CAD build for the part. Positions are in the model's coordinates, mm. Coordinates: 2 decimals unless noted, no trailing zeros. Loops run counter-clockwise (first coordinate to the right, second up) from the corner with the lowest first, then second, coordinate; pieces in that order, holes last. Notation, with made-up numbers: (33.5, 73) -> (79.5, 73) arc R31 ccw to (79.5, 102) -> close; hole circle Ø8 at (53.25, 36). An arc over 180 degrees is marked (long way). Answer as CSV lines item,"result". Start each with the question number.
from build123d import *

# Parameters (mm, degrees)
EXTRUDE_1_DEPTH = 7
EXTRUDE_2_DEPTH = 9


with BuildPart() as part:
    # 草图1 → 凸台-拉伸1 (new body)
    with BuildSketch(Plane(origin=(0, 0, 0), x_dir=(1, 0, 0), z_dir=(0, 1, 0))):
        Polygon((-112.559101124, 19.665498127), (-92.311400749, -15.404547658), (-72.063700375, -50.474593443), (-31.568299625, -50.474593443), (8.927101124, -50.474593443), (29.174801498, -15.404547658), (49.422501873, 19.665498127), (29.174801498, 54.735543912), (8.927101124, 89.805589698), (-31.568299625, 89.805589698), (-72.063700375, 89.805589698), (-92.311400749, 54.735543912), align=None)
        Polygon((-68.02224849, 86.805589698), (-34.455050971, 86.805589698), (-51.23864973, 57.735543912), align=None, mode=Mode.SUBTRACT)
        Polygon((8.349750855, 84.805589697), (24.555999345, 56.735543912), (-7.856497635, 56.735543912), align=None, mode=Mode.SUBTRACT)
        Polygon((-9.011198174, 52.735543912), (8.349750855, 22.665498127), (25.710699883, 52.735543912), align=None, mode=Mode.SUBTRACT)
        Polygon((28.597451229, 49.735543912), (44.803699719, 21.665498127), (12.39120274, 21.665498127), align=None, mode=Mode.SUBTRACT)
        Polygon((11.2365022, 17.665498127), (28.02010096, -11.404547658), (44.803699719, 17.665498127), align=None, mode=Mode.SUBTRACT)
        Polygon((-8.433847905, -16.404547658), (25.133349614, -16.404547658), (8.349750854, -45.474593443), align=None, mode=Mode.SUBTRACT)
        Polygon((-11.89794952, -18.404547658), (4.885649239, -47.474593443), (-28.68154828, -47.474593443), align=None, mode=Mode.SUBTRACT)
        Polygon((-28.681548279, 86.805589698), (4.885649241, 86.805589698), (-11.897949519, 57.735543911), align=None, mode=Mode.SUBTRACT)
        Polygon((-88.269948864, 55.735543912), (-71.486350105, 84.805589697), (-54.702751346, 55.735543912), align=None, mode=Mode.SUBTRACT)
        Polygon((-107.940298969, 21.665498127), (-91.15670021, 50.735543912), (-74.373101451, 21.665498127), align=None, mode=Mode.SUBTRACT)
        Polygon((-75.52780199, 17.665498127), (-107.94029897, 17.665498127), (-91.73405048, -10.404547658), align=None, mode=Mode.SUBTRACT)
        Polygon((-88.847299134, -13.404547658), (-54.125401077, -13.404547658), (-71.486350105, 16.665498127), align=None, mode=Mode.SUBTRACT)
        Polygon((-68.02224849, -47.474593443), (-34.455050971, -47.474593443), (-51.238649731, -18.404547658), align=None, mode=Mode.SUBTRACT)
        Polygon((-87.692598596, -17.404547658), (-71.486350105, -45.474593443), (-55.280101615, -17.404547658), align=None, mode=Mode.SUBTRACT)
    extrude(amount=EXTRUDE_1_DEPTH)

    # 草图2 → 凸台-拉伸2 (add)
    with BuildSketch(Plane(origin=(0, 7, 0), x_dir=(1, 0, 0), z_dir=(0, 1, 0))):
        Polygon((-71.486350105, 16.665498127), (-73.218400913, 19.665498127), (-52.393350269, 55.735543912), (-10.743248982, 55.735543912), (10.081801662, 19.665498127), (-10.743248982, -16.404547658), (-52.393350269, -16.404547658), align=None)
    extrude(amount=EXTRUDE_2_DEPTH)


solid = part.part
Item 1: Wall check: probe 1 along X at (y, z) = (1.25, 38); probe 2 along X at (y, z) = (1.75, 26); probe 3 along X at (y, z) = (6.75, 6). Give the ranges that are in metal, low to high.
Item 2: Flat gauge pins, fed straight in: pin 1 Ø2 at (x, y) = (34, 2) entering from -Z; pin 2 Ø6 at (y, z) = (5.5, -34) entering from -X; pin 3 Ø3.5 at (x, y) = (-80, 2.5) entering from -Z. Where does each tip first touch, or does it go through?
Item 3: Two-plate mould, pull along Z, no slides. Class faces 1 (the face through (-33, 0, -21)), 2 (the face through (-79.703, 3.451, 31.243)), 3 (the face through (-62.95, 11.44, -37.45)): pulls with the +Z half, pulls with the -Z half, needs draft (parallel to the pull), parting line crosses it, or undercut.
Item 4: Saw through at C-C (y = 12). Write the cut outline in (x, z), plus the area to 3 significant figures.
Item 5: Saw through at A-A (x = -18). Write the cut outline in (y, z).
Item 6: Saw through at D-D (x = -60.5). Write the cut outline in (y, z).
Item 7: Saw through at B-B (z = 0). Write the cut outline in (x, y).
Geometry check:
1,probe 1,"-79.27 to -75.8, -67.17 to -62.55, -39.93 to -23.21, -0.58 to 4.03, 12.67 to 16.13"
1,probe 2,"-86.19 to -82.73, -60.24 to -55.62, -46.85 to -16.28, -7.51 to -2.89, 19.59 to 23.06"
1,probe 3,"-97.74 to -94.28, -89.19 to -84.57, -58.4 to 24.9, 31.14 to 34.6"
2,pin 1,"z = -48.11"
2,pin 2,"x = -106.02"
2,pin 3,"z = -79.09"
3,face 1,"needs draft"
3,face 2,"undercut"
3,face 3,"pulls with the -Z half"
4,outline,"(-73.22, -19.67) -> (-52.39, -55.74) -> (-10.74, -55.74) -> (10.08, -19.67) -> (-10.74, 16.4) -> (-52.39, 16.4) -> close"
4,area,"4,510 mm2"
5,outline,"(0, -89.81) -> (7, -89.81) -> (7, -86.81) -> (0, -86.81) -> close; (0, -68.3) -> (7, -68.3) -> (7, -55.74) -> (16, -55.74) -> (16, 16.4) -> (7, 16.4) -> (7, 28.97) -> (0, 28.97) -> close; (0, 47.47) -> (7, 47.47) -> (7, 50.47) -> (0, 50.47) -> close"
6,outline,"(0, -89.81) -> (7, -89.81) -> (7, -86.81) -> (0, -86.81) -> close; (0, -73.78) -> (7, -73.78) -> (7, -65.78) -> (0, -65.78) -> close; (0, -55.74) -> (7, -55.74) -> (7, -41.69) -> (16, -41.69) -> (16, 2.36) -> (0, 2.36) -> close; (0, 13.4) -> (7, 13.4) -> (7, 17.4) -> (0, 17.4) -> close; (0, 26.45) -> (7, 26.45) -> (7, 34.45) -> (0, 34.45) -> close; (0, 47.47) -> (7, 47.47) -> (7, 50.47) -> (0, 50.47) -> close"
7,outline,"(-101.21, 0) -> (-97.74, 0) -> (-97.74, 7) -> (-101.21, 7) -> close; (-85.73, 0) -> (-81.11, 0) -> (-81.11, 7) -> (-85.73, 7) -> close; (-61.86, 0) -> (21.44, 0) -> (21.44, 7) -> (-1.27, 7) -> (-1.27, 16) -> (-61.86, 16) -> close; (34.6, 0) -> (38.07, 0) -> (38.07, 7) -> (34.6, 7) -> close"
